Answer from the drawing. Dimensions are ordinates in mm from the lowest x, y and z of the part. A direction names the side the tool comes from. Coordinates: 2 decimals unless noted, no trailing zeros. Write each loop counter-clockwise with the first axis right and the second up, starting at its lowest first coordinate (ties: lowest second). Pieces come first, ordered by that corner, then holes. Notation, with made-up numbers: (-8.5, 11.5) -> (5.5, 11.5) arc R28 cw to (5.5, 33.5) -> close; hole circle Ø9 at (2.25, 26). An arc over 180 degrees is marked (long way). Use CSV: the item, a comma, the result in double quotes.
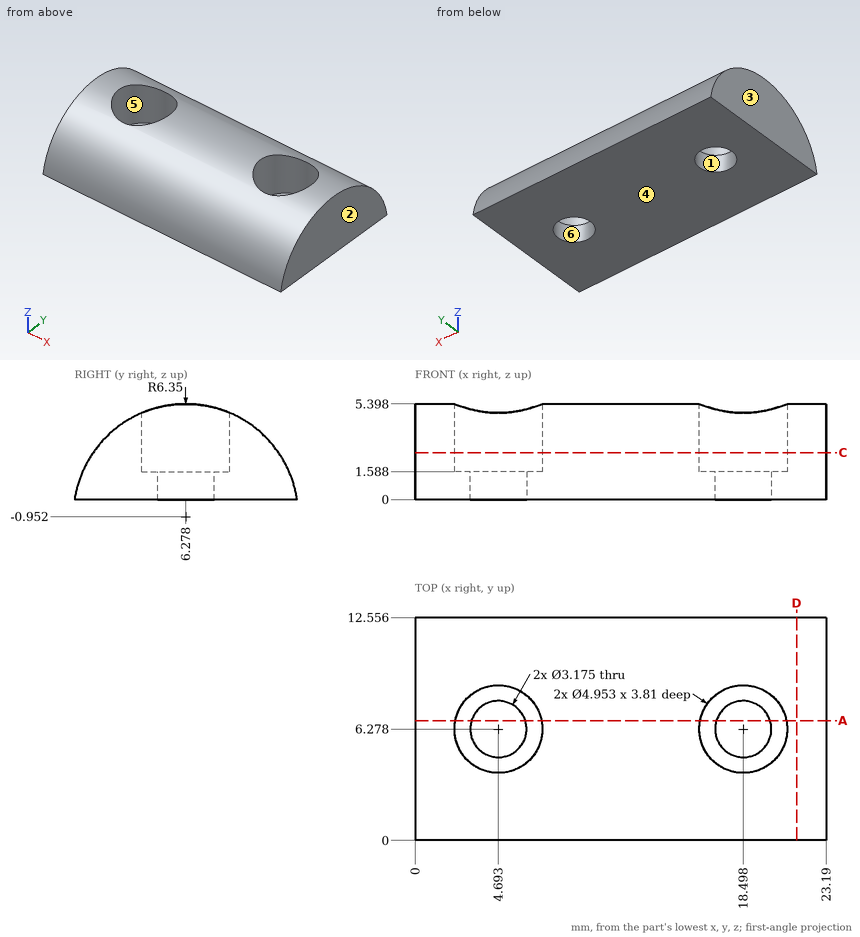
1. Each of these flat-tipped pins is pushed along its axis until it touches: pin 1 Ø3.5 at (x, y) = (4.69, 6.28) entering from -Z; pin 2 Ø4 at (x, y) = (4.5, 6.5) entering from +Z; pin 3 Ø2.5 at (x, y) = (18.5, 6.28) entering from +Z; pin 4 Ø2 at (x, z) = (20, 3.5) entering from -Y. Where does it stop, or does it pass through?
Solutions:
pin 1,"stops at z = 0"
pin 2,"stops at z = 1.59"
pin 3,"passes through"
pin 4,"stops at y = 0.95"
2. A cutting plane is placed at C-C (z = 2.65). Give the vertices of the cut face in (x, y) (1 decimal), and give its area (3 significant figures).
Solutions:
outline,"(0, 1) -> (23.2, 1) -> (23.2, 11.5) -> (0, 11.5) -> close; hole circle Ø5 at (4.7, 6.3); hole circle Ø5 at (18.5, 6.3)"
area,"204 mm^2"
3. A cutting plane is placed at D-D (x = 21.5). Give the vertices of the cut face in (y, z).
Solutions:
outline,"(0, 0) -> (12.56, 0) arc R6.35 ccw to start"
4. A cutting plane is placed at A-A (y = 6.75). Give the vertices of the cut face in (x, z).
Solutions:
outline,"(0, 0) -> (3.18, 0) -> (3.18, 1.59) -> (2.26, 1.59) -> (2.26, 5.38) -> (0, 5.38) -> close; (6.21, 0) -> (16.98, 0) -> (16.98, 1.59) -> (16.07, 1.59) -> (16.07, 5.38) -> (7.12, 5.38) -> (7.12, 1.59) -> (6.21, 1.59) -> close; (20.01, 0) -> (23.19, 0) -> (23.19, 5.38) -> (20.93, 5.38) -> (20.93, 1.59) -> (20.01, 1.59) -> close"
5. For a pull along X with two mould halves and no side action, classify the marked faces 1, 2, 3 and 4 as pulls with the +X half, pulls with the -X half, needs draft (parallel to the pull), parting line crosses it, or undercut.
Solutions:
face 1,"undercut"
face 2,"pulls with the +X half"
face 3,"pulls with the -X half"
face 4,"needs draft"
6. Find the intervals of material crossed by line 1 along X through (y, z) = (6, 1.5) (1 decimal); line 2 along X through (y, z) = (6, 3); line 3 along Z through (x, y) = (14.25, 6), in increasing order.
Solutions:
line 1,"x = 0 to 3.1, 6.3 to 16.9, 20.1 to 23.2"
line 2,"x = 0 to 2.23, 7.15 to 16.04, 20.96 to 23.19"
line 3,"z = 0 to 5.39"
7. A tool of negligible diameter and unlimited length cuts with its end or side. For the marked faces 5 and 6, from which of +Z, -Z, +X, -X, +Y, -Y can it reach the whole face along a straight path? Write none if from no direction.
Solutions:
face 5,"+Z"
face 6,"+Z, -Z"
